Geometry: final body of the model. Coordinates: model frame, mm. Face numbers are marked on the shaded views. A direction names the side the tool comes from. Give positions to 0.01 mm unless a question says otherwise; leave off trailing zeros. Write each loop counter-clockwise with the first axis right and the second up, starting at its lowest first coordinate (ties: lowest second). Pieces come first, ordered by that corner, then holes.
Q1. Section D-D (y = 55). Return the cut outline in (x, z), plus the area to 4 significant figures.
Q2. Pin query (flat end, axial travel): pin 1 Ø0.8 at (x, z) = (9, 1) entering from +Y; pin 2 Ø0.8 at (x, z) = (42.5, 1) entering from +Y; pin 3 Ø4 at (y, z) = (76.5, -8.5) entering from -X. Return the tip coordinate at first contact, or that it passes through.
Q3. Section A-A (x = 3.3). Return the cut outline in (y, z), plus the area to 3 significant figures.
Q4. Section C-C (x = 38). Return the cut outline in (y, z), plus the area to 3 significant figures.
Q5. Reachability of the marked faces 1 and 2 from +Z, -Z, +X, -X, +Y, -Y: full face, straight path, thin tool, end or side. Return the list, or none.
Q6. Section B-B (y = 3.8). Return the cut outline in (x, z).
Q7. Line query: line 1 (Y direction, x = 52.3, z = 0.5); line 2 (Y direction, x = 3.3, z = 0.45); line 3 (Y direction, x = 16, z = 0.5). Output: solid intervals per line, ascending.
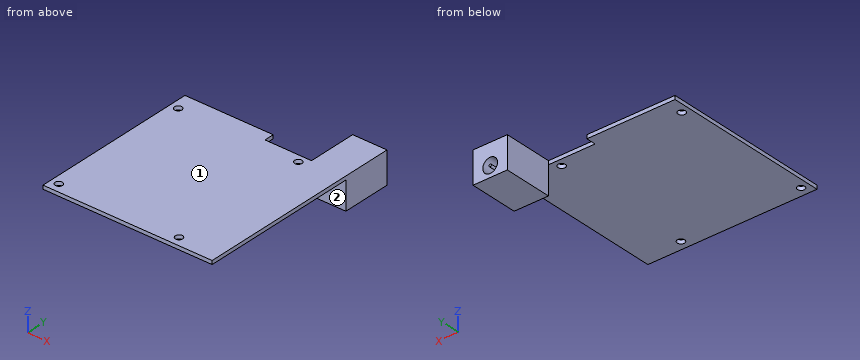
from build123d import *

# Parameters (mm, degrees)
SKETCH1_R           = 1.5
BOSS_EXTRUDE1_DEPTH = 1.5
SKETCH1_3_W         = 14
SKETCH1_3_H         = 20
BOSS_EXTRUDE2_DEPTH = 11.5
SKETCH2_R           = 3
SKETCH2_R_2         = 0.5
CUT_EXTRUDE1_DEPTH  = 10


with BuildPart() as part:
    # Sketch1 → Boss-Extrude1 (new body)
    with BuildSketch(Plane.XY):
        Polygon((55, 85), (55, 65), (36, 65), (36, 69), (0, 69), (0, 0), (69, 0), (69, 85), align=None)
        with Locations((52.3, 61.8)):
            Circle(SKETCH1_R, mode=Mode.SUBTRACT)
        with Locations((3.3, 3.8)):
            Circle(SKETCH1_R, mode=Mode.SUBTRACT)
        with Locations((52.3, 3.8)):
            Circle(SKETCH1_R, mode=Mode.SUBTRACT)
        with Locations((3.3, 61.8)):
            Circle(SKETCH1_R, mode=Mode.SUBTRACT)
    extrude(amount=BOSS_EXTRUDE1_DEPTH)

    # Sketch1_3 → Boss-Extrude2 (add)
    with BuildSketch(Plane.XY):
        with Locations((62, 75)):
            Rectangle(SKETCH1_3_W, SKETCH1_3_H)
    extrude(amount=-BOSS_EXTRUDE2_DEPTH)

    # Sketch2 → Cut-Extrude1 (cut)
    with BuildSketch(Plane(origin=(0, 85, 0), x_dir=(1, 0, 0), z_dir=(0, 1, 0))):
        with Locations(Location((62, 7, 0), (0, 0, 270))):  # turned: the seam where the file's is
            Circle(SKETCH2_R)
        with Locations(Location((62, 7, 0), (0, 0, 270))):  # turned: the seam where the file's is
            Circle(SKETCH2_R_2, mode=Mode.SUBTRACT)
    extrude(amount=-CUT_EXTRUDE1_DEPTH, mode=Mode.SUBTRACT)


solid = part.part
Computed:
1. outline: (0, 0) - (69, 0) - (69, 1.5) - (0, 1.5) - close
1. area: 103.5 mm2
2. pin 1: stops at y = 69
2. pin 2: stops at y = 65
2. pin 3: stops at x = 55
3. outline: (0, 0) - (2.3, 0) - (2.3, 1.5) - (0, 1.5) - close; (5.3, 0) - (60.3, 0) - (60.3, 1.5) - (5.3, 1.5) - close; (63.3, 0) - (69, 0) - (69, 1.5) - (63.3, 1.5) - close
3. area: 94.5 mm2
4. outline: (0, 0) - (65, 0) - (65, 1.5) - (0, 1.5) - close
4. area: 97.5 mm2
5. face 1: +Z, +X, -X, +Y, -Y
5. face 2: -Z, +X, -X, -Y
6. outline: (0, 0) - (1.8, 0) - (1.8, 1.5) - (0, 1.5) - close; (4.8, 0) - (50.8, 0) - (50.8, 1.5) - (4.8, 1.5) - close; (53.8, 0) - (69, 0) - (69, 1.5) - (53.8, 1.5) - close
7. line 1: y = 0 to 2.3, 5.3 to 60.3, 63.3 to 65
7. line 2: y = 0 to 2.3, 5.3 to 60.3, 63.3 to 69
7. line 3: y = 0 to 69
